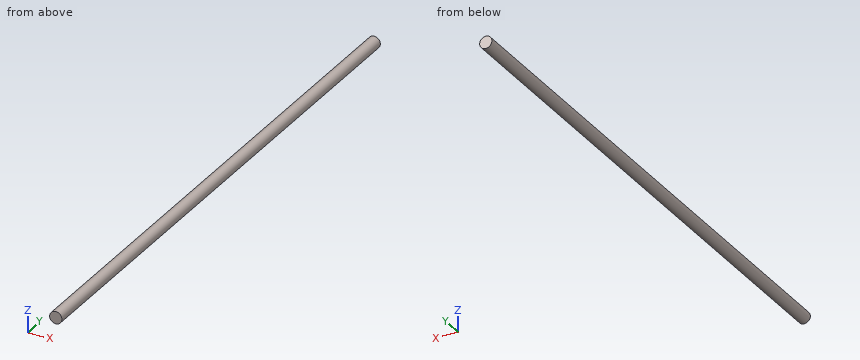
Autodesk Fusion 360 part; units mm, degrees
sketch "Sketch1" plane through (0, 0, 0) normal (0, 1, 0) x (1, 0, 0)
  circle A0 centre (0, 0) radius 3
  dimension "d1" = 6
extrude "Extrude1" add sketch "Sketch1" along normal blind 336
extrude "Extrude2" cut 1 faces at (-1.1591, 0, -0.5829) along direction (0, 1, 0) blind 50
extrude "Extrude3" cut 1 faces at (-1.1591, 50, -0.5829) along direction (0, 1, 0) blind 6
The listing builds one solid part. Answer for the finished solid, in the listing's coordinates (mm). Coordinates: 2 decimals unless noted, no trailing zeros. Order: outer loops, then holes, each group sorted by start corner. A loop starts at its lowest first (then second) coordinate and runs counter-clockwise, first axis right, second up. Notation, with made-up numbers: M -2.75,63.25 L 32.25,63.25 A7 cw 32.25,71.25 Z; hole C -13,73.5 d2. An arc over 180 degrees is marked long. Answer as a JSON object with one key per item and string values. Group by question number.
1. Flat-ended cylindrical pins translate along their axes: P1, Ø1.5, axis at x = 2, y = 162, coming from the +Z side; P2, Ø1, axis at x = 1, y = 226.5, coming from the -Z side; P3, Ø3, axis at y = 93, z = -2.5, coming from the +X side. Find the tip coordinate at first contact, or state that the pin passes through.
2. Section B-B on z = -1.85 is taken. Write down the section's boundary in (x, y), then the cut area to 3 significant figures.
3. Straight lines are drawn through the part: line 1 (Z direction, x = -0.3, y = 196); line 2 (Z direction, x = -0.55, y = 307); line 3 (X direction, y = 138.5, z = 0.7). For each, find the intervals that lie inside material, in ascending order.
4. Section C-C on x = 1.4 is taken. Write down the section's boundary in (y, z), then the cut area to 3 significant figures.
5. Section A-A on y = 302 is taken. Write down the section's boundary in (x, z), then the cut area to 3 significant figures.
Values follow:
{
 "1": {"P1": "z = 2.73", "P2": "z = -2.96", "P3": "x = 2.83"},
 "2": {"outline": "M -2.36,56 L 2.36,56 L 2.36,336 L -2.36,336 Z", "area": "1,320 mm2"},
 "3": {"line 1": "-2.98 to 2.98", "line 2": "-2.95 to 2.95", "line 3": "-2.92 to 2.92"},
 "4": {"outline": "M 56,-2.65 L 336,-2.65 L 336,2.65 L 56,2.65 Z", "area": "1,490 mm2"},
 "5": {"outline": "C 0,0 d6", "area": "28.3 mm2"}
}
